Part model, mm, in its own coordinate system. Coordinates: 2 decimals unless noted, no trailing zeros. Loops run counter-clockwise (first coordinate to the right, second up) from the corner with the lowest first, then second, coordinate; pieces in that order, holes last. Notation, with made-up numbers: (7.5, 27.25) - (60.5, 27.25) arc R26 cw to (60.5, 46.25) - close; hole circle Ø3 at (18, 71.25). An arc over 180 degrees is marked (long way). Use a Markdown table: item, result. Add a question column.
1) Pull direction Y, two halves, no side cores. Call faces 1 (the face through (0, 247, 127)), 2 (the face through (2.958, 128.745, 171.787)): +Y half, -Y half, draft (parallel to the pull), parting line (faces both ways), or undercut.
2) Band-saw the part on A-A (z = 147). Give the cut face in (x, y), plus the area to 3 significant figures.
3) Band-saw the part on C-C (x = 2.6). Give the cut face in (y, z), plus the area to 3 significant figures.
4) Probe probe 1 along Y at (x, z) = (2.1, 147.5) (3 decimals); probe 2 along Z at (x, y) = (3.4, 132); probe 3 along Y at (x, z) = (2.9, 139.5). List the from-to ranges inside material, lowest first. Write a range as [from, to].
5) Band-saw the part on B-B (y = 132). Give the cut face in (x, z), plus the area to 3 significant figures.
from build123d import *

# Parameters (mm, degrees)
SKETCH_W  = 500
SKETCH_H  = 250
SKETCH_R  = 25
PAD_DEPTH = 6


with BuildPart() as part:
    # Sketch → Pad (new body)
    with BuildSketch(Plane.YZ):
        with Locations((250, 125)):
            Rectangle(SKETCH_W, SKETCH_H)
        with Locations((132, 147)):
            Circle(SKETCH_R, mode=Mode.SUBTRACT)
    extrude(amount=PAD_DEPTH)


solid = part.part
Answer block:
| question | item | result |
|---|---|---|
| 1 | face 1 | draft |
| 1 | face 2 | undercut |
| 2 | outline | (0, 0) - (6, 0) - (6, 107) - (0, 107) - close; (0, 157) - (6, 157) - (6, 500) - (0, 500) - close |
| 2 | area | 2,700 mm2 |
| 3 | outline | (0, 0) - (500, 0) - (500, 250) - (0, 250) - close; hole circle Ø50 at (132, 147) |
| 3 | area | 123,000 mm2 |
| 4 | probe 1 | [0, 107.005], [156.995, 500] |
| 4 | probe 2 | [0, 122], [172, 250] |
| 4 | probe 3 | [0, 108.15], [155.85, 500] |
| 5 | outline | (0, 0) - (6, 0) - (6, 122) - (0, 122) - close; (0, 172) - (6, 172) - (6, 250) - (0, 250) - close |
| 5 | area | 1,200 mm2 |
